Here's how the part is built. I have some questions about the finished solid (model axes, mm). Round coordinates to 2 decimals unless told otherwise and drop trailing zeros. Write each loop counter-clockwise with the first axis right and the second up, starting at its lowest first coordinate (ties: lowest second). Pieces come first, ordered by that corner, then holes. Notation, with made-up numbers: (1.25, -35.5) -> (27.25, -35.5) arc R30 ccw to (27.25, -0.5) -> close; hole circle Ø7 at (72.25, 57). An arc over 180 degrees is marked (long way). Answer as CSV lines item,"result".
from build123d import *

# Parameters (mm, degrees)
BOX231_W          = 10
BOX231_H          = 10
BOX231_DEPTH      = 4
CYLINDER041_R     = 15
CYLINDER041_DEPTH = 32
BOX072_W          = 30
BOX072_H          = 6
BOX072_DEPTH      = 9


with BuildPart() as cube219:
    # Box231 → Box231 (new body)
    with BuildSketch(Plane(origin=(81, 40, -16), x_dir=(1, 0, 0), z_dir=(0, 0, 1))):
        with Locations((5, 5)):
            Rectangle(BOX231_W, BOX231_H)
    extrude(amount=BOX231_DEPTH)


with BuildPart() as cylinder128:
    # Cylinder041 → Cylinder041 (new body)
    with BuildSketch(Plane(origin=(0, 31, -15), x_dir=(0, 0, -1), z_dir=(1, 0, 0))):
        Circle(CYLINDER041_R)
    extrude(amount=CYLINDER041_DEPTH)


with BuildPart() as cut124:
    # Box072 → Box072 (new body)
    with BuildSketch(Plane(origin=(1, 40, -15), x_dir=(1, 0, 0), z_dir=(0, 0, 1))):
        with Locations((15, 3)):
            Rectangle(BOX072_W, BOX072_H)
    extrude(amount=BOX072_DEPTH)

    # Cut123: cut Cylinder128
    add(cylinder128.part, mode=Mode.SUBTRACT)


with BuildPart() as cut124_1:
    # Cut123 placement: moved
    add(cut124.part.moved(Location((87, 0, 0))))

    # Cut124: cut Cube219
    add(cube219.part, mode=Mode.SUBTRACT)


solid = cut124_1.part
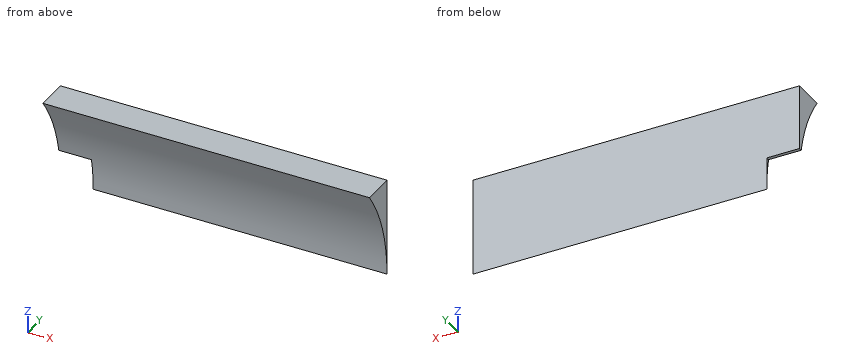
Item 1: Will this pin go through, and if not, where does the flat tip stop? pin 1 (5 mm diameter, centred on x = 100, z = -7, fed in from -Y).
Results found:
pin 1,"stops at y = 43"
Item 2: Suppose I cut it at A-A, the plane x = 97.5. List the corners of the cut face in (y, z) for me.
Results found:
outline,"(43, -6) arc R15 cw to (46, -15) -> (46, -6) -> close"
Item 3: I need wall thicknesses on L1, parallel to Y at x = 113.75, z = -7; L2, parallel to Z at x = 99, y = 43.3; L3, parallel to Z at x = 111, y = 44.3. Which ranges of each line are inside material? Lowest first, please.
Results found:
L1,"y = 43.69 to 46"
L2,"z = -6.41 to -6"
L3,"z = -8.06 to -6"
Item 4: Suppose I cut it at B-B, the plane z = -7. List the corners of the cut face in (x, y) for me, then the cut area to 3 significant figures.
Results found:
outline,"(88, 43.69) -> (118, 43.69) -> (118, 46) -> (88, 46) -> close"
area,"69.3 mm²"
Item 5: Suppose I cut it at C-C, the plane y = 44.6. List the corners of the cut face in (x, z) for me.
Results found:
outline,"(88, -8.67) -> (118, -8.67) -> (118, -6) -> (88, -6) -> close"
